Build history of the part. All positions in model axes, mm. A direction names the side the tool comes from. Give positions to 0.01 mm unless a question says otherwise; leave off trailing zeros. Write each loop counter-clockwise with the first axis right and the second up, starting at its lowest first coordinate (ties: lowest second). Pieces come first, ordered by that corner, then holes.
from build123d import *

# Parameters (mm, degrees)
SKETCH3_R           = 2.07
BOSS_EXTRUDE1_DEPTH = 1.5
FILLET1_R           = 3


with BuildPart() as part:
    # Sketch3 → Boss-Extrude1 (new, symmetric)
    with BuildSketch(Plane.XY):
        Polygon((0, 0), (0, -101.6), (50.8, -101.6), (50.8, -63.5), (101.6, -50.8), (101.6, 0), (50.8, 0), align=None)
        with Locations((12.7, -88.9)):
            Circle(SKETCH3_R, mode=Mode.SUBTRACT)
        with Locations((12.7, -63.5)):
            Circle(SKETCH3_R, mode=Mode.SUBTRACT)
        with Locations((12.7, -38.1)):
            Circle(SKETCH3_R, mode=Mode.SUBTRACT)
        with Locations((12.7, -12.7)):
            Circle(SKETCH3_R, mode=Mode.SUBTRACT)
        with Locations(Location((38.1, -12.7, 0), (0, 0, 180))):
            Circle(SKETCH3_R, mode=Mode.SUBTRACT)
        with Locations(Location((38.1, -38.1, 0), (0, 0, 180))):
            Circle(SKETCH3_R, mode=Mode.SUBTRACT)
        with Locations(Location((38.1, -63.5, 0), (0, 0, 180))):
            Circle(SKETCH3_R, mode=Mode.SUBTRACT)
        with Locations(Location((38.1, -88.9, 0), (0, 0, 180))):
            Circle(SKETCH3_R, mode=Mode.SUBTRACT)
        with Locations((25.4, -76.2)):
            Circle(SKETCH3_R, mode=Mode.SUBTRACT)
        with Locations((25.4, -63.5)):
            Circle(SKETCH3_R, mode=Mode.SUBTRACT)
        with Locations((25.4, -50.8)):
            Circle(SKETCH3_R, mode=Mode.SUBTRACT)
        with Locations((25.4, -38.1)):
            Circle(SKETCH3_R, mode=Mode.SUBTRACT)
        with Locations((25.4, -25.4)):
            Circle(SKETCH3_R, mode=Mode.SUBTRACT)
        with Locations(Location((50.8, -12.7, 0), (0, 0, 180))):
            Circle(SKETCH3_R, mode=Mode.SUBTRACT)
        with Locations(Location((50.8, -38.1, 0), (0, 0, 180))):
            Circle(SKETCH3_R, mode=Mode.SUBTRACT)
        with Locations(Location((63.5, -12.7, 0), (0, 0, 180))):
            Circle(SKETCH3_R, mode=Mode.SUBTRACT)
        with Locations(Location((63.5, -38.1, 0), (0, 0, 180))):
            Circle(SKETCH3_R, mode=Mode.SUBTRACT)
        with Locations(Location((76.2, -12.7, 0), (0, 0, 180))):
            Circle(SKETCH3_R, mode=Mode.SUBTRACT)
        with Locations(Location((76.2, -38.1, 0), (0, 0, 180))):
            Circle(SKETCH3_R, mode=Mode.SUBTRACT)
        with Locations(Location((88.9, -12.7, 0), (0, 0, 180))):
            Circle(SKETCH3_R, mode=Mode.SUBTRACT)
        with Locations(Location((88.9, -38.1, 0), (0, 0, 180))):
            Circle(SKETCH3_R, mode=Mode.SUBTRACT)
        with Locations((50.8, -25.4)):
            Circle(SKETCH3_R, mode=Mode.SUBTRACT)
        with Locations((76.2, -25.4)):
            Circle(SKETCH3_R, mode=Mode.SUBTRACT)
    extrude(amount=BOSS_EXTRUDE1_DEPTH, both=True)

    # Fillet1
    fillet1_edges = [part.edges().sort_by_distance(p)[0] for p in [
        (101.6, 0, 0),
        (101.6, -50.8, 0),
        (50.8, -63.5, 0),
        (50.8, -101.6, 0),
        (0, -101.6, 0),
        (0, 0, 0),
    ]]
    fillet(fillet1_edges, radius=FILLET1_R)


solid = part.part
(1) Mould opens along Y. For faces 1 (the face through (51.453, -63.974, 0.021)), 2 (the face through (100.7, -0.86, -0.02)), 3 (the face through (90.97, -12.79, -0.02)), 4 (the face through (101.6, -26, 0)) say: +Y half, -Y half, draft (parallel to the pull), parting line (faces both ways), or undercut.
(2) Saw through at B-B, the plane y = -38.1. Give the number of separate pieces and of enclosed holes in the cut face, plus the area to 3 significant figures.
(3) Saw through at D-D, the plane x = 63.5. List the corners of the cut face in (y, z) (3 decimals).
(4) Saw through at C-C, the plane y = -25.4. List the corners of the cut face in (x, z), plus the area to 3 significant figures.
(5) Saw through at A-A, the plane x = 25.4. List the corners of the cut face in (y, z).
(6) 3-axis set-ups, long thin cutter, end or side, ignore diameter. For faces 5 (the face through (50.8, -82, 0)), 6 (the face through (61.526, -13.322, -0.021)): which of +Z, -Z, +X, -X, +Y, -Y reach the whole face in a straight line?
(7) Probe line 1 (Y direction, x = 25.4, z = 0.9); line 2 (Y direction, x = 12.7, z = 0.7); line 3 (Y direction, x = 88, z = 0.1). List the from-to ranges inside material, lowest first.
(8) Drop a flat-ended pin along its axis: pin 1 (1.5 mm diameter, centred on y = -80.5, z = 0, fed in from +X). Give the stop position or say it passes through.
Computed values:
1. face 1: -Y half
1. face 2: +Y half
1. face 3: undercut
1. face 4: draft
2. separate pieces: 8
2. enclosed holes: 0
2. area: 218 mm2
3. outline: (-60.325, -1.5) - (-40.17, -1.5) - (-40.17, 1.5) - (-60.325, 1.5) - close; (-36.03, -1.5) - (-14.77, -1.5) - (-14.77, 1.5) - (-36.03, 1.5) - close; (-10.63, -1.5) - (0, -1.5) - (0, 1.5) - (-10.63, 1.5) - close
4. outline: (0, -1.5) - (23.33, -1.5) - (23.33, 1.5) - (0, 1.5) - close; (27.47, -1.5) - (48.73, -1.5) - (48.73, 1.5) - (27.47, 1.5) - close; (52.87, -1.5) - (74.13, -1.5) - (74.13, 1.5) - (52.87, 1.5) - close; (78.27, -1.5) - (101.6, -1.5) - (101.6, 1.5) - (78.27, 1.5) - close
4. area: 268 mm2
5. outline: (-101.6, -1.5) - (-78.27, -1.5) - (-78.27, 1.5) - (-101.6, 1.5) - close; (-74.13, -1.5) - (-65.57, -1.5) - (-65.57, 1.5) - (-74.13, 1.5) - close; (-61.43, -1.5) - (-52.87, -1.5) - (-52.87, 1.5) - (-61.43, 1.5) - close; (-48.73, -1.5) - (-40.17, -1.5) - (-40.17, 1.5) - (-48.73, 1.5) - close; (-36.03, -1.5) - (-27.47, -1.5) - (-27.47, 1.5) - (-36.03, 1.5) - close; (-23.33, -1.5) - (0, -1.5) - (0, 1.5) - (-23.33, 1.5) - close
6. face 5: +Z, -Z, +X, -Y
6. face 6: +Z, -Z
7. line 1: y = -101.6 to -78.27, -74.13 to -65.57, -61.43 to -52.87, -48.73 to -40.17, -36.03 to -27.47, -23.33 to 0
7. line 2: y = -101.6 to -90.97, -86.83 to -65.57, -61.43 to -40.17, -36.03 to -14.77, -10.63 to 0
7. line 3: y = -54.2 to -39.96, -36.24 to -14.56, -10.84 to 0
8. pin 1: stops at x = 50.8
